Work out the finished part from the listing and answer in its coordinate system (mm). Coordinates: 2 decimals unless noted, no trailing zeros. Loops run counter-clockwise (first coordinate to the right, second up) from the corner with the lowest first, then second, coordinate; pieces in that order, holes last.
```python
from build123d import *

# Parameters (mm, degrees)
F1_W     = 1500
F1_H     = 12
F2_DEPTH = 225
F4_DEPTH = 225


with BuildPart() as f2:
    # F1 (on Front) → F2 (new body, symmetric)
    with BuildSketch(Plane.XZ):
        with Locations((0, 344)):
            Rectangle(F1_W, F1_H)
    extrude(amount=F2_DEPTH, both=True)

    # F3 (on face) → F4 (join, through all)
    with BuildSketch(Plane.XZ):
        Polygon((-648.1164097786, 338), (-750, 338), (-699.4419693947, 248), (-648.1164097786, 248), (-648.1164097786, 282.9072217941), align=None)
    extrude(amount=F4_DEPTH)


solid = f2.part
```
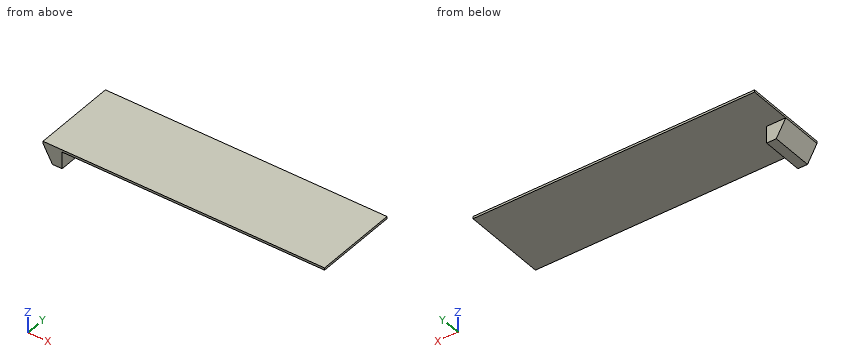
1. Each of these flat-tipped pins is pushed along its axis until it touches: P1, Ø1.5, axis at y = -43, z = 259, coming from the +X side; P2, Ø3, axis at x = -384, y = -117, coming from the -Z side. Where does it stop, or does it pass through?
2. Straight lines are drawn through the part: probe 1 along Z at (x, y) = (639.5, -127.5); probe 2 along X at (y, z) = (-70, 297.5); probe 3 along X at (y, z) = (-0.5, 275.5). For each, find the intervals that lie inside material, in ascending order.
3. A cutting plane is placed at C-C, the plane z = 307.5. Give the vertices of the cut face in (x, y).
4. A cutting plane is placed at A-A, the plane y = -98. Give the vertices of the cut face in (x, z).
5. A cutting plane is placed at B-B, the plane x = 453.5. Give the vertices of the cut face in (y, z).
Answers below:
1. P1: stops at x = -648.12
1. P2: stops at z = 338
2. probe 1: z = 338 to 350
2. probe 2: x = -727.25 to -648.12
2. probe 3: x = -714.89 to -648.12
3. outline: (-732.87, -225) - (-648.12, -225) - (-648.12, 0) - (-732.87, 0) - close
4. outline: (-750, 338) - (-699.44, 248) - (-648.12, 248) - (-648.12, 338) - (750, 338) - (750, 350) - (-750, 350) - close
5. outline: (-225, 338) - (225, 338) - (225, 350) - (-225, 350) - close
